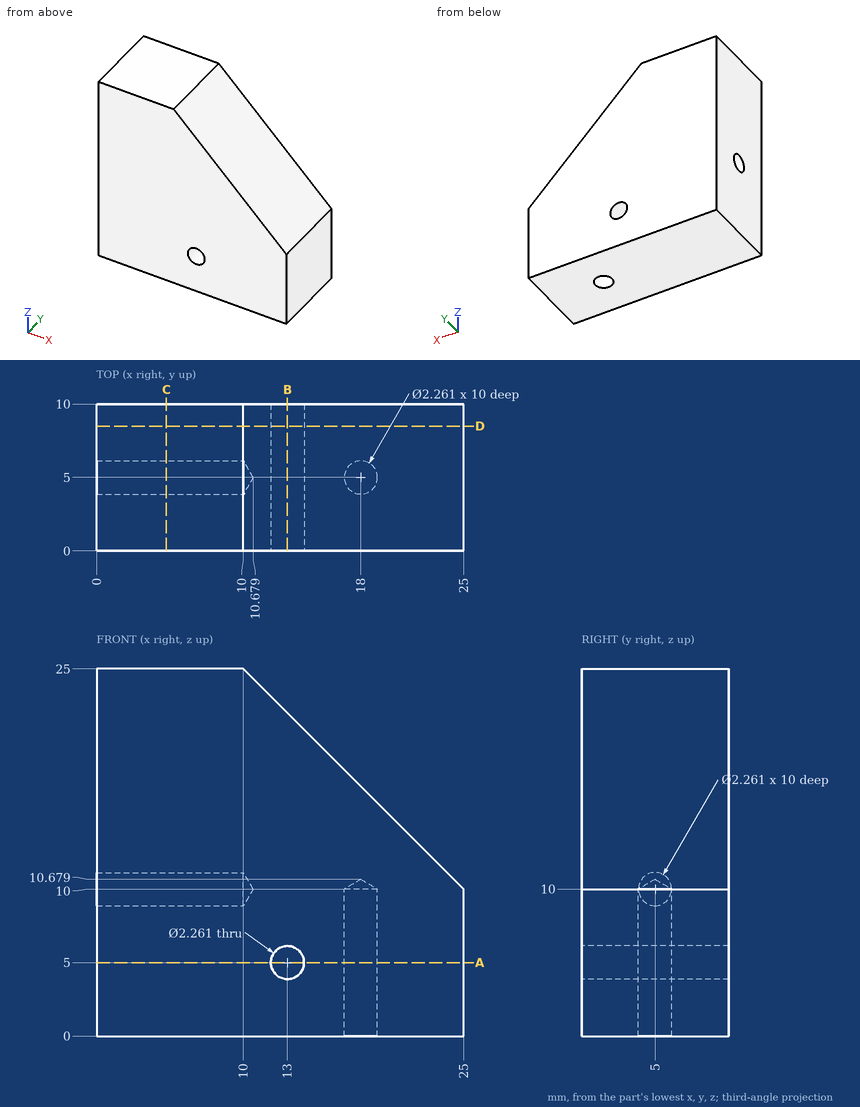
Geometry: see drawing. Coordinates: mm, zero at the bounding-box minimum. Coordinates: 2 decimals unless noted, no trailing zeros. Order: outer loops, then holes, each group sorted by start corner. A loop starts at its lowest first (then second) coordinate and runs counter-clockwise, first axis right, second up. Notation, with made-up numbers: M 29,63 L 71,63 A9 cw 71,69 Z; hole C 17,19 d9. An arc over 180 degrees is marked long. Write item = value, one per line. Start each with the question number.
(1) Section D-D on y = 8.5. Output: boundary loops of the cut face in (x, z).
(2) Section A-A on z = 5. Output: boundary loops of the cut face in (x, y), and give its area (3 significant figures).
(3) Section C-C on x = 4.75. Output: boundary loops of the cut face in (y, z).
(4) Section B-B on x = 13. Output: boundary loops of the cut face in (y, z), and give its area (3 significant figures).
(5) First-contact query: P1, Ø4, axis at y = 7, z = 17, coming from the +X side; P2, Ø1.4, axis at x = 13, z = 5, coming from the +Y side; P3, Ø2, axis at y = 5, z = 10, coming from the -X side. Flat tips, straight axial feed; report the tip coordinate or a pass-through.
(6) Line query: line 1 along Y through (x, z) = (18, 2.75); line 2 along Z through (x, y) = (2.25, 5); line 3 along X through (y, z) = (7.25, 5). Output: solid intervals per line, ascending. Write a range as [from, to].
Result set:
q1.outline = M 0,0 L 25,0 L 25,10 L 10,25 L 0,25 Z; hole C 13,5 d2.26
q2.outline = M 0,0 L 11.87,0 L 11.87,10 L 0,10 Z; M 14.13,0 L 25,0 L 25,10 L 14.13,10 Z; hole C 18,5 d2.26
q2.area = 223 mm²
q3.outline = M 0,0 L 10,0 L 10,25 L 0,25 Z; hole C 5,10 d2.26
q4.outline = M 0,0 L 10,0 L 10,3.87 L 0,3.87 Z; M 0,6.13 L 10,6.13 L 10,22 L 0,22 Z
q4.area = 197 mm²
q5.P1 = 20
q5.P2 = through
q5.P3 = 10.08
q6.line_1 = [0, 3.87], [6.13, 10]
q6.line_2 = [0, 8.87], [11.13, 25]
q6.line_3 = [0, 11.87], [14.13, 25]
